For this review, take the finished solid that the model builds, in its own axes (mm). A direction names the side the tool comes from. Coordinates: 2 decimals unless noted, no trailing zeros. Loops run counter-clockwise (first coordinate to the right, second up) from the corner with the lowest first, then second, coordinate; pieces in that order, holes last. Notation, with made-up numbers: (33, -24) - (52, -24) arc R13 ccw to (52, -15) - close; hole circle Ø3 at (6.25, 23). An arc over 180 degrees is marked (long way). Use one line per item in the form item = value. Start each with the question number.
1. To check wall thickness, follow probe 1 along Z at (x, y) = (5.75, 0.2); probe 2 along X at (y, z) = (1.55, 1.85); probe 3 along Z at (x, y) = (4.5, 0.8). State the ranges of each line that lie inside material, in increasing order.
2. Add section C-C on y = 1.1. Give the boundary of the cut face in (x, z).
3. Add section B-B on x = 6. Give the boundary of the cut face in (y, z).
4. Draft analysis for pull direction X (two halves, no side actions). For faces 1 (the face through (6.5, 1, 2)), 2 (the face through (4, 1, 4)), 3 (the face through (8, 1, 2)), state which applies: +X half, -X half, draft (parallel to the pull), parting line (faces both ways), or undercut.
5. Add section D-D on x = 3. Give the boundary of the cut face in (y, z).
6. Add section A-A on z = 1.4. Give the boundary of the cut face in (x, y), and give its area (3 significant figures).
7. Machinability: for faces 4 (the face through (4.953, 1, 0.5)), 5 (the face through (2, 1, 1)), 6 (the face through (3.9, 0, 3.4)), which of the approach directions +Z, -Z, +X, -X, +Y, -Y give a long, thin tool a straight path to every point of the face, cutting with its end or side? Answer none if there is none.
```python
from build123d import *

# Parameters (mm, degrees)
F1_DEPTH = 2
F2_DEPTH = 25


with BuildPart() as f1:
    # F0 (on Front) → F1 (new body)
    with BuildSketch(Plane.XZ):
        Polygon((0, 4), (0, 0), (2.890676, 0), (2.890676, 1), (1.5, 1), (1.5, 3), (6.5, 3), (6.5, 1), (4.952536, 1), (4.952536, 0), (8, 0), (8, 4), align=None)
        Polygon((2.890676, 1), (2.890676, 0), (4.952536, 0), (4.952536, 1), (6.5, 1), (6.5, 3), (1.5, 3), (1.5, 1), align=None)
    extrude(amount=-F1_DEPTH)

    # F0 (on Front) → F2 (cut)
    with BuildSketch(Plane.XZ):
        Polygon((2.890676, 1), (2.890676, 0), (4.952536, 0), (4.952536, 1), (6.5, 1), (6.5, 3), (1.5, 3), (1.5, 1), align=None)
    extrude(amount=-F2_DEPTH, mode=Mode.SUBTRACT)


solid = f1.part
```
Conclusion:
q1.probe_1 = 0 to 1, 3 to 4
q1.probe_2 = 0 to 1.5, 6.5 to 8
q1.probe_3 = 3 to 4
q2.outline = (0, 0) - (2.89, 0) - (2.89, 1) - (1.5, 1) - (1.5, 3) - (6.5, 3) - (6.5, 1) - (4.95, 1) - (4.95, 0) - (8, 0) - (8, 4) - (0, 4) - close
q3.outline = (0, 0) - (2, 0) - (2, 1) - (0, 1) - close; (0, 3) - (2, 3) - (2, 4) - (0, 4) - close
q4.face_1 = undercut
q4.face_2 = draft
q4.face_3 = +X half
q5.outline = (0, 3) - (2, 3) - (2, 4) - (0, 4) - close
q6.outline = (0, 0) - (1.5, 0) - (1.5, 2) - (0, 2) - close; (6.5, 0) - (8, 0) - (8, 2) - (6.5, 2) - close
q6.area = 6.00 mm^2
q7.face_4 = -Z, +Y, -Y
q7.face_5 = +Y, -Y
q7.face_6 = +Z, -Z, +X, -X, -Y
